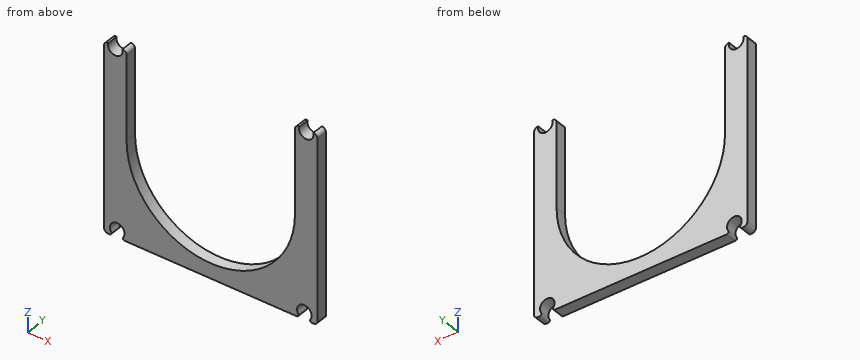
```python
from build123d import *

# Parameters (mm, degrees)
F1_DEPTH = 6
F2_R     = 3.9
F3_DEPTH = 6.001
F4_R     = 2
F5_R     = 1


with BuildPart() as f1:
    # F0 (on Front) → F1 (new body)
    with BuildSketch(Plane.XZ):
        with BuildLine():
            ThreePointArc((45, 53), (0, 8), (-45, 53))
            Line((-45, 53), (-45, 100))
            Line((-45, 100), (-47.230384635, 100))
            ThreePointArc((-47.230384635, 100), (-51, 95.1), (-54.769615365, 100))
            Line((-54.769615365, 100), (-57, 100))
            Line((-57, 100), (-57, 0))
            Line((-57, 0), (57, 0))
            Line((57, 0), (57, 100))
            Line((57, 100), (54.769615365, 100))
            ThreePointArc((54.769615365, 100), (51, 95.1), (47.230384635, 100))
            Line((47.230384635, 100), (45, 100))
            Line((45, 100), (45, 53))
        make_face()
    extrude(amount=F1_DEPTH)

    # F2 (on Front) → F3 (cut, through all)
    with BuildSketch(Plane.XZ):
        with Locations((-50, 3.7)):
            Circle(F2_R)
        with Locations((50, 3.7)):
            Circle(F2_R)
    extrude(amount=F3_DEPTH, mode=Mode.SUBTRACT)

    # F4
    f4_edges = [f1.edges().sort_by_distance(p)[0] for p in [
        (-45, -3, 100),
        (45, -3, 100),
        (-57, -3, 100),
        (57, -3, 100),
        (57, -3, 0),
        (-57, -3, 0),
    ]]
    fillet(f4_edges, radius=F4_R)

    # F5
    f5_edges = [f1.edges().sort_by_distance(p)[0] for p in [
        (-48.767117, -3, 0),
        (-51.232883, -3, 0),
        (51.232883, -3, 0),
        (48.767117, -3, 0),
    ]]
    fillet(f5_edges, radius=F5_R)


solid = f1.part
```
The model under review builds one solid part; all positions refer to its coordinate system, in mm. Give positions to 0.01 mm unless a question says otherwise; leave off trailing zeros. Write each loop counter-clockwise with the first axis right and the second up, starting at its lowest first coordinate (ties: lowest second). Pieces come first, ordered by that corner, then holes. Notation, with made-up numbers: (17.25, 7) -> (76.25, 7) arc R29 cw to (76.25, 28) -> close; hole circle Ø4 at (-35, 13). An arc over 180 degrees is marked (long way). Put each result on its own line as item: value.
(1) We need section B-B, the plane y = -3.6. Give the boundary of the cut face in (x, z).
Results are:
outline: (-57, 2) arc R2 ccw to (-55, 0) -> (-54.09, 0) arc R1 ccw to (-53.25, 1.55) arc R3.9 cw (long way) to (-46.75, 1.55) arc R1 ccw to (-45.91, 0) -> (45.91, 0) arc R1 ccw to (46.75, 1.55) arc R3.9 cw (long way) to (53.25, 1.55) arc R1 ccw to (54.09, 0) -> (55, 0) arc R2 ccw to (57, 2) -> (57, 98) arc R2 ccw to (55, 100) -> (54.77, 100) arc R3.9 cw (long way) to (47.23, 100) -> (47, 100) arc R2 ccw to (45, 98) -> (45, 53) arc R45 cw to (-45, 53) -> (-45, 98) arc R2 ccw to (-47, 100) -> (-47.23, 100) arc R3.9 cw (long way) to (-54.77, 100) -> (-55, 100) arc R2 ccw to (-57, 98) -> close
(2) We need section C-C, the plane x = 14. Give the boundary of the cut face in (y, z).
Results are:
outline: (-6, 0) -> (0, 0) -> (0, 10.23) -> (-6, 10.23) -> close
(3) To check wall thickness, follow probe 1 along X at (y, z) = (-1.2, 3.7); probe 2 along X at (y, z) = (-0.55, 62); probe 3 along X at (y, z) = (-1.45, 99). State the ranges of each line that lie inside material, in increasing order. Write a range as from..to.
Results are:
probe 1: -57..-53.9, -46.1..46.1, 53.9..57
probe 2: -57..-45, 45..57
probe 3: -56.73..-54.9, -47.1..-45.27, 45.27..47.1, 54.9..56.73
(4) We need section A-A, the plane x = 0. Give the boundary of the cut face in (y, z), and give its area (3 significant figures).
Results are:
outline: (-6, 0) -> (0, 0) -> (0, 8) -> (-6, 8) -> close
area: 48.0 mm²
(5) For pin 1 Ø2 at (x, y) = (-1.5, -5.5) entering from +Z, flat-tipped, find the tip position at first contact; note if it passes through.
Results are:
pin 1: z = 8.07
